Verification items for the finished model (mm, model axes). A direction names the side the tool comes from. Round coordinates to 2 decimals unless told otherwise and drop trailing zeros. Loops run counter-clockwise (first coordinate to the right, second up) from the corner with the lowest first, then second, coordinate; pieces in that order, holes last. Notation, with made-up numbers: M 50.5,8.25 L 61.5,8.25 A15 cw 61.5,32.25 Z; hole C -23.5,61 d5. An arc over 180 degrees is marked long. One line per item, written item: value.
from build123d import *

# Parameters (mm, degrees)
SKETCH1_R           = 22.225
SKETCH1_R_2         = 12.7
SKETCH1_R_3         = 2.5781
BOSS_EXTRUDE1_DEPTH = 44.45
SKETCH2_R           = 6.35
CUT_EXTRUDE1_DEPTH  = 44.45


with BuildPart() as part:
    # Sketch1 → Boss-Extrude1 (new body)
    with BuildSketch(Plane.XY):
        Circle(SKETCH1_R)
        Circle(SKETCH1_R_2, mode=Mode.SUBTRACT)
        with Locations((0, 17.81175)):
            Circle(SKETCH1_R_3, mode=Mode.SUBTRACT)
        with Locations((0, -17.907)):
            Circle(SKETCH1_R_3, mode=Mode.SUBTRACT)
    extrude(amount=BOSS_EXTRUDE1_DEPTH)

    # Sketch2 → Cut-Extrude1 (cut)
    with BuildSketch(Plane(origin=(0, 0, 0), x_dir=(0, 0, -1), z_dir=(1, 0, 0))):
        with Locations((-8.89, 0)):
            Circle(SKETCH2_R)
    extrude(amount=-CUT_EXTRUDE1_DEPTH, mode=Mode.SUBTRACT)


solid = part.part
(1) Sectioned sample at C-C on y = -12. Enter the section's corners in (x, z).
Completed:
outline: M -18.71,0 L -4.16,0 L -4.16,44.45 L -18.71,44.45 Z; M 4.16,0 L 18.71,0 L 18.71,44.45 L 4.16,44.45 Z
(2) Sectioned sample at B-B on x = 0. Enter the section's corners in (y, z) (3 decimals).
Completed:
outline: M -22.225,0 L -20.485,0 L -20.485,44.45 L -22.225,44.45 Z; M -15.329,0 L -12.7,0 L -12.7,44.45 L -15.329,44.45 Z; M 12.7,0 L 15.234,0 L 15.234,44.45 L 12.7,44.45 Z; M 20.39,0 L 22.225,0 L 22.225,44.45 L 20.39,44.45 Z
(3) Tool access check on faces 1 (the face through (-0.559, -20.424, 21.914)), 2 (the face through (-16.533, 5.354, 5.476)). Record the directions out of +Z, -Z, +X, -X, +Y, -Y that give a thin tool (end or side, any length) a straight path to the whole face; none if there is none.
Completed:
face 1: +Z, -Z
face 2: -X
(4) Sectioned sample at D-D on x = -6.5. Enter the section's corners in (y, z), and give its area (3 significant figures).
Completed:
outline: M -21.25,0 L -10.91,0 L -10.91,44.45 L -21.25,44.45 Z; M 10.91,0 L 21.25,0 L 21.25,44.45 L 10.91,44.45 Z
area: 919 mm^2
(5) Mould release check, pull along Y, two halves, no side actions. Record for faces 3 (the face through (10, -10, 44.45)), 4 (the face through (21.199, 6.676, 21.914)), 5 (the face through (12.114, 3.815, 21.914)): +Y half, -Y half, draft (parallel to the pull), parting line (faces both ways), or undercut.
Completed:
face 3: draft
face 4: parting line
face 5: undercut
(6) Depth check by flat-ended pin: pin 1 Ø1.5 at (x, y) = (5.5, -14.5) entering from -Z; pin 2 Ø1.5 at (y, z) = (6, 38) entering from -X; pin 3 Ø10 at (x, z) = (-5.5, 20.5) entering from +Y; pin 4 Ø3 at (x, y) = (0, 17.81) entering from +Z. Enter the tip coordinate at first touch or a pass-through.
Completed:
pin 1: stops at z = 0
pin 2: stops at x = -21.6
pin 3: stops at y = 22.22
pin 4: passes through
(7) Thickness scan on L1, parallel to Y at x = 0, z = 33 (3 decimals); L2, parallel to X at y = 0, z = 35 (3 decimals); L3, parallel to X at y = 6.5, z = 18.5. Record the ranges inside material, lowest first. Write a range as from..to.
Completed:
L1: y = -22.225..-20.485, -15.329..-12.7, 12.7..15.234, 20.39..22.225
L2: x = -22.225..-12.7, 12.7..22.225
L3: x = -21.25..-10.91, 10.91..21.25
(8) Sectioned sample at A-A on y = 0. Enter the section's corners in (x, z) (3 decimals), and give its area (3 significant figures).
Completed:
outline: M -22.225,0 L -12.7,0 L -12.7,2.54 L -22.225,2.54 Z; M -22.225,15.24 L -12.7,15.24 L -12.7,44.45 L -22.225,44.45 Z; M 12.7,0 L 22.225,0 L 22.225,44.45 L 12.7,44.45 Z
area: 726 mm^2
